from build123d import *

# Parameters (mm, degrees)
SKETCH1_R           = 7.65
SKETCH1_R_2         = 5.1
BOSS_EXTRUDE1_DEPTH = 0.6


with BuildPart() as part:
    # Sketch1 → Boss-Extrude1 (new body)
    with BuildSketch(Plane.XY):
        Circle(SKETCH1_R)
        Circle(SKETCH1_R_2, mode=Mode.SUBTRACT)
        with BuildLine():
            ThreePointArc((0, 5.6), (0.8, 6.4), (0, 7.2))
            ThreePointArc((0, 7.2), (-1.404650319, 7.061654019), (-2.755320713, 6.651932634))
            ThreePointArc((-2.755320713, 6.651932634), (-3.188277593, 5.606682262), (-2.143027221, 5.173725382))
            ThreePointArc((-2.143027221, 5.173725382), (-1.092505803, 5.49239757), (0, 5.6))
        make_face(mode=Mode.SUBTRACT)
        with BuildLine():
            ThreePointArc((6.651932634, 2.755320713), (5.606682262, 3.188277593), (5.173725382, 2.143027221))
            ThreePointArc((5.173725382, 2.143027221), (5.49239757, 1.092505803), (5.6, 0))
            ThreePointArc((5.6, 0), (6.4, -0.8), (7.2, 0))
            ThreePointArc((7.2, 0), (7.061654019, 1.404650319), (6.651932634, 2.755320713))
        make_face(mode=Mode.SUBTRACT)
        with BuildLine():
            ThreePointArc((2.755320713, -6.651932634), (3.188277593, -5.606682262), (2.143027221, -5.173725382))
            ThreePointArc((2.143027221, -5.173725382), (1.092505803, -5.49239757), (0, -5.6))
            ThreePointArc((0, -5.6), (-0.8, -6.4), (0, -7.2))
            ThreePointArc((0, -7.2), (1.404650319, -7.061654019), (2.755320713, -6.651932634))
        make_face(mode=Mode.SUBTRACT)
        with BuildLine():
            ThreePointArc((-6.651932634, -2.755320713), (-5.606682262, -3.188277593), (-5.173725382, -2.143027221))
            ThreePointArc((-5.173725382, -2.143027221), (-5.49239757, -1.092505803), (-5.6, 0))
            ThreePointArc((-5.6, 0), (-6.4, 0.8), (-7.2, 0))
            ThreePointArc((-7.2, 0), (-7.061654019, -1.404650319), (-6.651932634, -2.755320713))
        make_face(mode=Mode.SUBTRACT)
    extrude(amount=BOSS_EXTRUDE1_DEPTH)


solid = part.part
Work out the finished part from the listing and answer in its coordinate system (mm). Coordinates: 2 decimals unless noted, no trailing zeros. Write each loop counter-clockwise with the first axis right and the second up, starting at its lowest first coordinate (ties: lowest second). Pieces come first, ordered by that corner, then holes. Notation, with made-up numbers: M 24.5,-27 L 76.5,-27 A31 ccw 76.5,7 Z; hole C -25,73.5 d9. An arc over 180 degrees is marked long. Answer as CSV lines item,"result". Start each with the question number.
Item 1: Section A-A on y = 4.25 is taken. Write down the section's boundary in (x, z), and give its area (3 significant figures).
Item 2: Section C-C on x = -6.25 is taken. Write down the section's boundary in (y, z).
Item 3: A flat-ended cylindrical pin translates along its axis: P1, Ø6, axis at x = -5.5, y = -5.5, coming from the -Z side. Find the tip coordinate at first contact, or state that the pin passes through.
Item 4: Section D-D on x = 2.5 is taken. Write down the section's boundary in (y, z), and give its area (3 significant figures).
Item 5: Consider L1, parallel to Y at x = -2.75, z = 0.45; L2, parallel to Y at x = -1.25, z = 0.3; L3, parallel to X at y = -1, z = 0.25. Determine where each line is inside the solid, lowest interval first.
Item 6: Determine the mould class of faces 1 (the face through (3.195, -5.623, 0.296)), 2 (the face through (5.623, 3.195, 0.296)), 3 (the face through (2, -5, 0)), 4 (the face through (-1.658, -7.468, 0.296)) for opening direction X: released by +X, released by -X, zero draft, split by the parting line, or undercut.
Item 7: Section B-B on z = 0.5 is taken. Write down the section's boundary in (x, y), and give its area (3 significant figures).
Checks:
1,outline,"M -6.36,0 L -2.82,0 L -2.82,0.6 L -6.36,0.6 Z; M 2.82,0 L 6.36,0 L 6.36,0.6 L 2.82,0.6 Z"
1,area,"4.25 mm²"
2,outline,"M -4.41,0 L -3.17,0 L -3.17,0.6 L -4.41,0.6 Z; M 0.79,0 L 4.41,0 L 4.41,0.6 L 0.79,0.6 Z"
3,P1,"stops at z = 0"
4,outline,"M -7.23,0 L -6.75,0 L -6.75,0.6 L -7.23,0.6 Z; M -5.11,0 L -4.45,0 L -4.45,0.6 L -5.11,0.6 Z; M 4.45,0 L 7.23,0 L 7.23,0.6 L 4.45,0.6 Z"
4,area,"2.36 mm²"
5,L1,"y = -7.14 to -4.3, 4.3 to 5.17, 6.65 to 7.14"
5,L2,"y = -7.55 to -4.94, 4.94 to 5.46, 7.09 to 7.55"
5,L3,"x = -7.58 to -7.13, -5.51 to -5, 5 to 7.58"
6,face 1,"undercut"
6,face 2,"undercut"
6,face 3,"zero draft"
6,face 4,"split by the parting line"
7,outline,"C 0,0 d15.3; hole M -7.2,0 A7.2 ccw -6.65,-2.76 A0.8 ccw -5.17,-2.14 A5.6 cw -5.6,0 A0.8 ccw Z; hole C 0,0 d10.2; hole M -2.76,6.65 A0.8 ccw -2.14,5.17 A5.6 cw 0,5.6 A0.8 ccw 0,7.2 A7.2 ccw Z; hole M 0,-7.2 A7.2 ccw 2.76,-6.65 A0.8 ccw 2.14,-5.17 A5.6 cw 0,-5.6 A0.8 ccw Z; hole M 5.17,2.14 A5.6 cw 5.6,0 A0.8 ccw 7.2,0 A7.2 ccw 6.65,2.76 A0.8 ccw Z"
7,area,"78.0 mm²"
